Check sheet for the modelled part. Datum: model origin and axes. Units: mm. A direction names the side the tool comes from. Give positions to 0.01 mm unless a question says otherwise; leave off trailing zeros. Write each loop counter-clockwise with the first axis right and the second up, starting at its lowest first coordinate (ties: lowest second). Pieces come first, ordered by that corner, then holes. Notation, with made-up numbers: M -18.75,85.5 L -13.75,85.5 A15 cw -13.75,99.5 Z; hole C -0.5,22.5 d7. An arc over 180 degrees is marked long. Write each question's results on one line, items separated by ' | '. Start each with the question number.
Autodesk Inventor part; units mm, degrees
ref_plane "YZ Plane" through (0, 0, 0) normal (1, 0, 0) x (0, 1, 0)
ref_plane "XZ Plane" through (0, 0, 0) normal (0, 1, 0) x (-1, 0, 0)
ref_plane "XY Plane" through (0, 0, 0) normal (0, 0, 1) x (1, 0, 0)
sketch "Sketch1" plane through (0, 0, 0) normal (0, 0, 1) x (1, 0, 0)
  circle A0 centre (0, 0) radius 10
  circle A1 centre (0, 0) radius 15
  circle A2 centre (0, 0) radius 20
  line L0 (-20, 0) -> (20, 0)
  line L1 (20, 0) -> (20, -50)
  line L2 (20, -50) -> (-20, -50)
  line L3 (-20, -50) -> (-20, 0)
  line L4 (-20, -40) -> (20, -40)
  line L5 (20, -40) -> (20, -50)
  line L6 (20, -50) -> (-20, -50)
  line L7 (-20, -50) -> (-20, -40)
  line L8 (-5, -13) -> (5, -13)
  line L9 (5, -13) -> (5, -40)
  line L10 (5, -40) -> (-5, -40)
  line L11 (-5, -40) -> (-5, -13)
  point P0 (0, -50)
  point P1 (0, -40)
  dimension "d0" = 20
  dimension "d1" = 30
  dimension "d2" = 40
  dimension "d3" = 40
  dimension "d4" = 50
  dimension "d5" = 40
  dimension "d6" = 10
  dimension "d7" = 10
  dimension "d8" = 27
extrude "Extrusion1" add sketch "Sketch1" along normal blind 35 contours L0 A1 L9 L8 L11 A0 | A0 L0 A1 | L9 A2 L11 A1 | A1 L11 L8 L9 | L9 L4 L11 A2
extrude "Extrusion2" add sketch "Sketch1" along normal blind 10 contours L0 A0 | L0 A1 L9 L8 L11 A0 | A0 L0 | L0 A2 L9 A1 | A1 L0 A2 | A1 L11 A2 L0 | L9 A2 L11 A1 | L1 L4 L9 A2 | A2 L11 L4 L3
extrude "Extrusion3" add sketch "Sketch1" along normal blind 60 contours L1 L2 L3 L4
properties part number "A"
Q1. Depth check by flat-ended pin: pin 1 Ø6 at (x, y) = (1.5, 5) entering from +Z; pin 2 Ø6 at (x, z) = (2, 37) entering from +Y; pin 3 Ø8 at (x, y) = (11.5, 11.5) entering from +Z. Enter the tip coordinate at first touch or a pass-through.
Q2. Tool access check on faces 5 (the face through (-0.59, 14.99, 22.32)), 6 (the face through (0, -45, 60)), 7 (the face through (0, -50, 30)), 8 (the face through (5, -27, 22)), 9 (the face through (-5, -27, 22)). Record the directions out of +Z, -Z, +X, -X, +Y, -Y that give a thin tool (end or side, any length) a straight path to the whole face; none if there is none.
Q3. Section check B-B on x = 0. Record the boundary of the cut face in (y, z), plus the area to 4 significant figures.
Q4. Section check D-D on z = 6. Record the boundary of the cut face in (x, y).
Q5. Section check A-A on z = 13. Record the boundary of the cut face in (x, y), plus the area to 3 significant figures.
Q6. Scan lines: L1, parallel to Y at x = 0, z = 23; L2, parallel to Y at x = 2.5, z = 41; L3, parallel to Z at x = 2.5, y = 17. Record each from-to range of solid material in increasing order.
Q7. Release check for a two-part mould opening along X. For faces 1 (the face through (0, 0, 10)), 2 (the face through (-2.17, 9.76, 22.32)), 3 (the face through (0, 20, 5)), 4 (the face through (0, -12, 35)) record: pulls with the +X half, pulls with the -X half, needs draft (parallel to the pull), parting line crosses it, or undercut.
Q8. Section check C-C on y = -12.5. Record the boundary of the cut face in (x, z).
Check result:
1) pin 1: z = 10 | pin 2: y = 15 | pin 3: z = 35
2) face 5: +Z | face 6: +Z, +X, -X, +Y, -Y | face 7: +Z, -Z, +X, -X, -Y | face 8: +Z, +X | face 9: +Z, -X
3) outline: M -50,0 L 20,0 L 20,10 L 15,10 L 15,35 L 10,35 L 10,10 L -10,10 L -10,35 L -40,35 L -40,60 L -50,60 Z | area: 2,075 mm^2
4) outline: M -20,-50 L 20,-50 L 20,0 A20 ccw -20,0 Z
5) outline: M -20,-50 L 20,-50 L 20,-40 L 5,-40 L 5,-14.14 A15 ccw long -5,-14.14 L -5,-40 L -20,-40 Z; hole C 0,0 d20 | area: 1,050 mm^2
6) L1: -50 to -10, 10 to 15 | L2: -50 to -40 | L3: 0 to 10
7) face 1: undercut | face 2: undercut | face 3: parting line crosses it | face 4: needs draft
8) outline: M -20,0 L 20,0 L 20,10 L 8.29,10 L 8.29,35 L -8.29,35 L -8.29,10 L -20,10 Z
